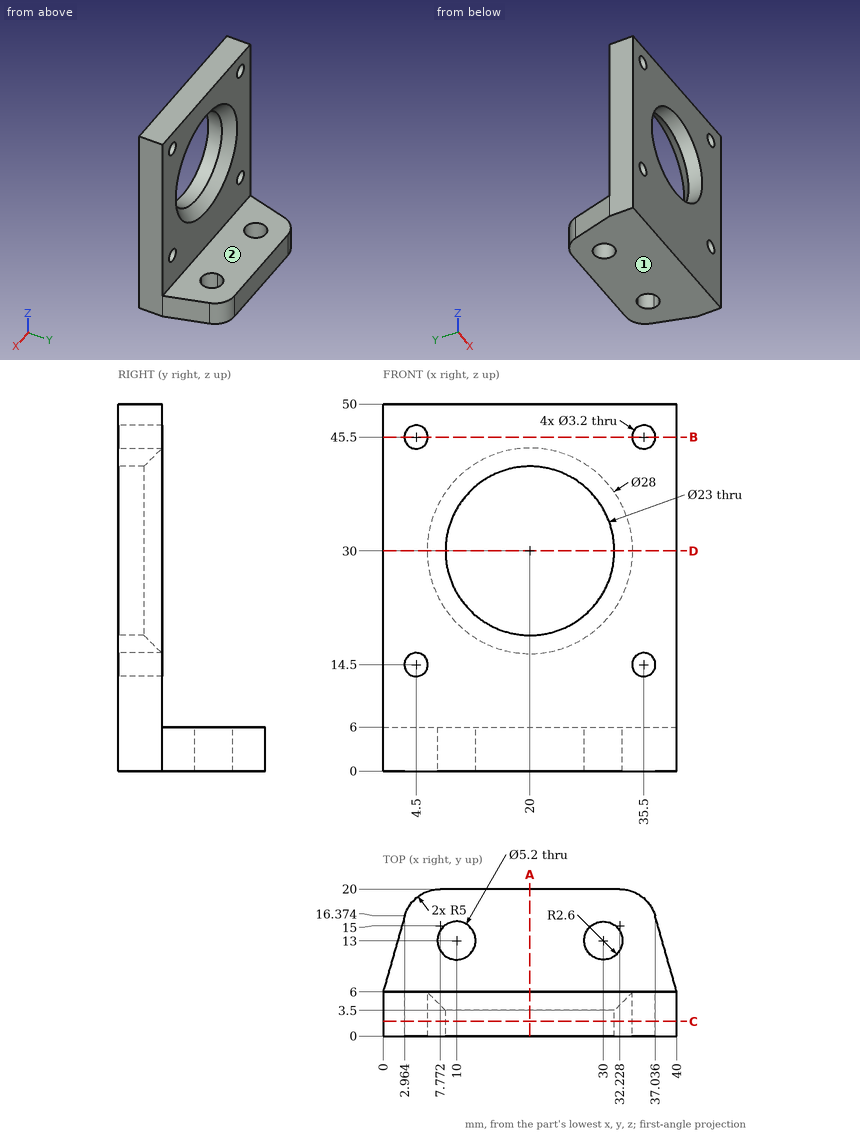
Could you check a few things on this drawing? It's one solid part, dimensions in mm from its lowest x, y, z. A direction names the side the tool comes from. Give positions to 0.01 mm unless a question says otherwise; leave off trailing zeros. Write each loop counter-clockwise with the first axis right and the second up, starting at its lowest first coordinate (ties: lowest second). Pieces come first, ordered by that corner, then holes. Notation, with made-up numbers: (59, -2.5) - (64, -2.5) arc R26 cw to (64, 30.5) - close; hole circle Ø2 at (1, -15). An arc over 180 degrees is marked (long way). Use CSV: the item, a comma, the result in double quotes. Start each with the question number.
Item 1: I want a section at A-A, the plane x = 20. Please give me the cut outline in (y, z), then the cut area to 3 significant figures.
Item 2: I want a section at C-C, the plane y = 2. Please give me the cut outline in (x, z).
Item 3: If I drill on line 1 along Z through (x, y) = (35.5, 3.2); line 2 along Z through (x, y) = (20, 1.55); line 3 along Z through (x, y) = (32, 17), over which ranges is the centre line in solid material (lowest first)?
Item 4: I'm going to push flat-ended pins straight in: pin 1 (7 mm diameter, centred on x = 10, y = 11.5, fed in from +Z); pin 2 (2 mm diameter, centred on x = 18, z = 18, fed in from +Y) (1 decimal). Where does each tip first touch, or does it pass through?
Item 5: For the marked faces 1 and 2, which set-ups out of +Z, -Z, +X, -X, +Y, -Y let a thin tool reach every point of the face, with its end or its side?
Item 6: I want a section at D-D, the plane z = 30. Please give me the cut outline in (x, y).
Item 7: I want a section at B-B, the plane z = 45.5. Please give me the cut outline in (x, y).
Findings:
1,outline,"(0, 0) - (20, 0) - (20, 6) - (6, 6) - (6, 16) - (3.5, 18.5) - (0, 18.5) - close; (0, 41.5) - (3.5, 41.5) - (6, 44) - (6, 50) - (0, 50) - close"
1,area,"240 mm2"
2,outline,"(0, 0) - (40, 0) - (40, 50) - (0, 50) - close; hole circle Ø3.2 at (4.5, 14.5); hole circle Ø3.2 at (4.5, 45.5); hole circle Ø23 at (20, 30); hole circle Ø3.2 at (35.5, 14.5); hole circle Ø3.2 at (35.5, 45.5)"
3,line 1,"z = 0 to 12.9, 16.1 to 43.9, 47.1 to 50"
3,line 2,"z = 0 to 18.5, 41.5 to 50"
3,line 3,"z = 0 to 6"
4,pin 1,"stops at z = 6"
4,pin 2,"stops at y = 5.2"
5,face 1,"-Z, +X, -X, +Y, -Y"
5,face 2,"+Z, +X, -X, +Y"
6,outline,"(0, 0) - (8.5, 0) - (8.5, 3.5) - (6, 6) - (0, 6) - close; (31.5, 0) - (40, 0) - (40, 6) - (34, 6) - (31.5, 3.5) - close"
7,outline,"(0, 0) - (2.9, 0) - (2.9, 6) - (0, 6) - close; (6.1, 0) - (33.9, 0) - (33.9, 6) - (6.1, 6) - close; (37.1, 0) - (40, 0) - (40, 6) - (37.1, 6) - close"
